Work out the finished part from the listing and answer in its coordinate system (mm). Give positions to 0.01 mm unless a question says otherwise; leave off trailing zeros. Loops run counter-clockwise (first coordinate to the right, second up) from the corner with the lowest first, then second, coordinate; pieces in that order, holes last. Notation, with made-up numbers: (23, 17) - (36, 17) arc R13 cw to (36, 40) - close; hole circle Ø8 at (-13.75, -39). An arc over 180 degrees is marked (long way). One line per item, written item: value.
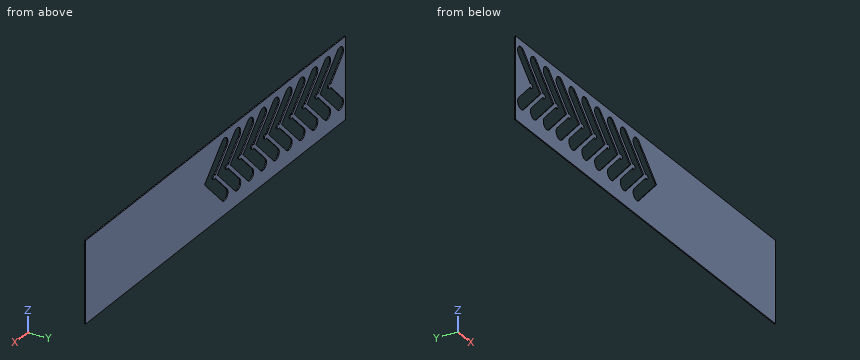
from build123d import *

# Parameters (mm, degrees)
SKETCH1_W           = 202.358038397
SKETCH1_H           = 38.375945136
BOSS_EXTRUDE1_DEPTH = 0.5


with BuildPart() as part:
    # Sketch1 → Boss-Extrude1 (new body)
    with BuildSketch(Plane(origin=(0, 0, 0), x_dir=(1, 0, 0), z_dir=(0, 1, 0))):
        with Locations((64.252599363, 1.75)):
            Rectangle(SKETCH1_W, SKETCH1_H)
        with BuildLine():
            Line((-34.635608145, 9.828784258), (-25.513930667, 0.707106781))
            ThreePointArc((-25.513930667, 0.707106781), (-23.806823886, 0), (-25.513930667, -0.707106781))
            Line((-25.513930667, -0.707106781), (-34.635608145, -9.828784258))
            ThreePointArc((-34.635608145, -9.828784258), (-34.635608145, -13.647160877), (-30.817231526, -13.647160877))
            Line((-30.817231526, -13.647160877), (-17.170070649, 0))
            Line((-17.170070649, 0), (-30.817231526, 13.647160877))
            ThreePointArc((-30.817231526, 13.647160877), (-34.635608145, 13.647160877), (-34.635608145, 9.828784258))
        make_face(mode=Mode.SUBTRACT)
        with BuildLine():
            Line((-20.817231526, 13.647160877), (-7.170070649, 0))
            Line((-7.170070649, 0), (-20.817231526, -13.647160877))
            ThreePointArc((-20.817231526, -13.647160877), (-24.635608145, -13.647160877), (-24.635608145, -9.828784258))
            Line((-24.635608145, -9.828784258), (-15.513930667, -0.707106781))
            ThreePointArc((-15.513930667, -0.707106781), (-13.806823886, 0), (-15.513930667, 0.707106781))
            Line((-15.513930667, 0.707106781), (-24.635608145, 9.828784258))
            ThreePointArc((-24.635608145, 9.828784258), (-24.635608145, 13.647160877), (-20.817231526, 13.647160877))
        make_face(mode=Mode.SUBTRACT)
        with BuildLine():
            Line((-10.817231526, 13.647160877), (2.829929351, 0))
            Line((2.829929351, 0), (-10.817231526, -13.647160877))
            ThreePointArc((-10.817231526, -13.647160877), (-14.635608145, -13.647160877), (-14.635608145, -9.828784258))
            Line((-14.635608145, -9.828784258), (-5.513930667, -0.707106781))
            ThreePointArc((-5.513930667, -0.707106781), (-3.806823886, 0), (-5.513930667, 0.707106781))
            Line((-5.513930667, 0.707106781), (-14.635608145, 9.828784258))
            ThreePointArc((-14.635608145, 9.828784258), (-14.635608145, 13.647160877), (-10.817231526, 13.647160877))
        make_face(mode=Mode.SUBTRACT)
        with BuildLine():
            Line((-0.817231526, 13.647160877), (12.829929351, 0))
            Line((12.829929351, 0), (-0.817231526, -13.647160877))
            ThreePointArc((-0.817231526, -13.647160877), (-4.635608145, -13.647160877), (-4.635608145, -9.828784258))
            Line((-4.635608145, -9.828784258), (4.486069333, -0.707106781))
            ThreePointArc((4.486069333, -0.707106781), (6.193176114, 0), (4.486069333, 0.707106781))
            Line((4.486069333, 0.707106781), (-4.635608145, 9.828784258))
            ThreePointArc((-4.635608145, 9.828784258), (-4.635608145, 13.647160877), (-0.817231526, 13.647160877))
        make_face(mode=Mode.SUBTRACT)
        with BuildLine():
            Line((9.182768474, 13.647160877), (22.829929351, 0))
            Line((22.829929351, 0), (9.182768474, -13.647160877))
            ThreePointArc((9.182768474, -13.647160877), (5.364391855, -13.647160877), (5.364391855, -9.828784258))
            Line((5.364391855, -9.828784258), (14.486069333, -0.707106781))
            ThreePointArc((14.486069333, -0.707106781), (16.193176114, 0), (14.486069333, 0.707106781))
            Line((14.486069333, 0.707106781), (5.364391855, 9.828784258))
            ThreePointArc((5.364391855, 9.828784258), (5.364391855, 13.647160877), (9.182768474, 13.647160877))
        make_face(mode=Mode.SUBTRACT)
        with BuildLine():
            Line((19.182768474, 13.647160877), (32.829929351, 0))
            Line((32.829929351, 0), (19.182768474, -13.647160877))
            ThreePointArc((19.182768474, -13.647160877), (15.364391855, -13.647160877), (15.364391855, -9.828784258))
            Line((15.364391855, -9.828784258), (24.486069333, -0.707106781))
            ThreePointArc((24.486069333, -0.707106781), (26.193176114, 0), (24.486069333, 0.707106781))
            Line((24.486069333, 0.707106781), (15.364391855, 9.828784258))
            ThreePointArc((15.364391855, 9.828784258), (15.364391855, 13.647160877), (19.182768474, 13.647160877))
        make_face(mode=Mode.SUBTRACT)
        with BuildLine():
            Line((29.182768474, 13.647160877), (42.829929351, 0))
            Line((42.829929351, 0), (29.182768474, -13.647160877))
            ThreePointArc((29.182768474, -13.647160877), (25.364391855, -13.647160877), (25.364391855, -9.828784258))
            Line((25.364391855, -9.828784258), (34.486069333, -0.707106781))
            ThreePointArc((34.486069333, -0.707106781), (36.193176114, 0), (34.486069333, 0.707106781))
            Line((34.486069333, 0.707106781), (25.364391855, 9.828784258))
            ThreePointArc((25.364391855, 9.828784258), (25.364391855, 13.647160877), (29.182768474, 13.647160877))
        make_face(mode=Mode.SUBTRACT)
        with BuildLine():
            Line((39.182768474, 13.647160877), (52.829929351, 0))
            Line((52.829929351, 0), (39.182768474, -13.647160877))
            ThreePointArc((39.182768474, -13.647160877), (35.364391855, -13.647160877), (35.364391855, -9.828784258))
            Line((35.364391855, -9.828784258), (44.486069333, -0.707106781))
            ThreePointArc((44.486069333, -0.707106781), (46.193176114, 0), (44.486069333, 0.707106781))
            Line((44.486069333, 0.707106781), (35.364391855, 9.828784258))
            ThreePointArc((35.364391855, 9.828784258), (35.364391855, 13.647160877), (39.182768474, 13.647160877))
        make_face(mode=Mode.SUBTRACT)
        with BuildLine():
            Line((49.182768474, 13.647160877), (62.829929351, 0))
            Line((62.829929351, 0), (49.182768474, -13.647160877))
            ThreePointArc((49.182768474, -13.647160877), (45.364391855, -13.647160877), (45.364391855, -9.828784258))
            Line((45.364391855, -9.828784258), (54.486069333, -0.707106781))
            ThreePointArc((54.486069333, -0.707106781), (56.193176114, 0), (54.486069333, 0.707106781))
            Line((54.486069333, 0.707106781), (45.364391855, 9.828784258))
            ThreePointArc((45.364391855, 9.828784258), (45.364391855, 13.647160877), (49.182768474, 13.647160877))
        make_face(mode=Mode.SUBTRACT)
        with BuildLine():
            Line((59.182768474, 13.647160877), (72.829929351, 0))
            Line((72.829929351, 0), (59.182768474, -13.647160877))
            ThreePointArc((59.182768474, -13.647160877), (55.364391855, -13.647160877), (55.364391855, -9.828784258))
            Line((55.364391855, -9.828784258), (64.486069333, -0.707106781))
            ThreePointArc((64.486069333, -0.707106781), (66.193176114, 0), (64.486069333, 0.707106781))
            Line((64.486069333, 0.707106781), (55.364391855, 9.828784258))
            ThreePointArc((55.364391855, 9.828784258), (55.364391855, 13.647160877), (59.182768474, 13.647160877))
        make_face(mode=Mode.SUBTRACT)
    extrude(amount=BOSS_EXTRUDE1_DEPTH)


solid = part.part
1. Find the intervals of material crossed by line 1 along Z through (x, y) = (-26, 0.45); line 2 along Z through (x, y) = (55, 0.25); line 3 along Z through (x, y) = (-2.5, 0.4), in increasing order.
Output:
line 1: z = -20.94 to -8.83, -1.19 to 1.19, 8.83 to 17.44
line 2: z = -20.94 to -13.19, -10.28 to -7.83, -0.98 to 0.98, 7.83 to 10.28, 13.19 to 17.44
line 3: z = -20.94 to -14.43, -7.69 to -5.33, 5.33 to 7.69, 14.43 to 17.44
2. Section B-B (y = 0.25) is taken. Count the separate pieces of the cut face and the enclosed holes in it, and give its area (3 significant figures).
Output:
separate pieces: 1
enclosed holes: 10
area: 5,770 mm²
3. Section A-A (x = 71) is taken. Write down the section's boundary in (y, z).
Output:
outline: (0, -20.94) - (0.5, -20.94) - (0.5, -1.83) - (0, -1.83) - close; (0, 1.83) - (0.5, 1.83) - (0.5, 17.44) - (0, 17.44) - close
